Autodesk Fusion 360 part; units mm, degrees
sketch "Sketch1" plane through (0, 0, 0) normal (0, 0, 1) x (1, 0, 0)
  circle A0 centre (0, 0) radius 5.45
  line L0 (0, 7.5) -> (0, -6)
  line L1 (-1.5, 5.2395) -> (-1.5, 3.45)
  line L2 (-1.5, 3.45) -> (1.5, 3.45)
  line L3 (1.5, 3.45) -> (1.5, 5.2395)
  circle A1 centre (0, 0) radius 3.2
  line L4 (-2.0805, -2.4314) -> (2.0805, -2.4314)
  point P0 (0, 5.45)
  dimension "d1" = 10.9
  dimension "d2" = 2
  dimension "d3" = 3
  dimension "d4" = 6.4
  dimension "d5" = 4.161
extrude "Extrude1" add sketch "Sketch1" along normal blind 15
extrude "Extrude2" add sketch "Sketch1" against normal blind 12 contours A0 L0 L2 L3 A1 | A0 L0 L2 L3 | A0 L0 L1 L2 A1 | A0 L0 L1 L2 | L0 A1 L4 | L0 A1 L4 picked at (-0.1505, -2.9331) picked at (0.1518, 1.312)
extrude "Extrude3" cut sketch "Sketch1" against normal blind 10 from surface at 15 contours A0 L0 L2 L3 | A0 L0 L1 L2
Geometry check sheet. Reference: the model listing, model coordinates, mm. A direction names the side the tool comes from. Give positions to 0.01 mm unless a question says otherwise; leave off trailing zeros. Order: outer loops, then holes, each group sorted by start corner. A loop starts at its lowest first (then second) coordinate and runs counter-clockwise, first axis right, second up. Notation, with made-up numbers: (-4.5, 75.5) - (6.5, 75.5) arc R15 ccw to (6.5, 79.5) - close; hole circle Ø8 at (2, 65.5). An arc over 180 degrees is marked (long way). Write item = value, one per line. Start each with the question number.
1) Draft check along Y on faces 4 (the cylindrical face through (-2.982, 1.16, -5.916)), 5 (the flat face through (1, 0, -12)), 6 (the flat face through (0, 3.45, 10)), 7 (the flat face through (-1, 0, 0)). Enter one of: released by +Y, released by -Y, zero draft, split by the parting line, or undercut.
2) Scan lines: L1, parallel to X at y = 0, z = -4; L2, parallel to Z at x = 1, y = -2.5; L3, parallel to Y at x = 1.25, z = -7.5. Record each from-to range of solid material in increasing order.
3) Section check A-A (y = 0). Enter the section's corners in (x, z).
4) Section check D-D (x = 3.25). Enter the section's corners in (y, z), then the cut area to 3 significant figures.
5) Gauge pin test, flat ends, axial feed: pin 1 Ø2.5 at (x, z) = (1.5, -5) entering from -Y; pin 2 Ø1.5 at (y, z) = (4, 10.5) entering from -X; pin 3 Ø1.6 at (x, y) = (0.5, 4.5) entering from +Z. Record the tip position at first contact, or that the pin passes through.
6) Access from +Z, -Z, +X, -X, +Y, -Y to the whole of each face (thin tool, end or side, straight path). Record for faces 1 (the cylindrical face through (2.515, -4.835, 1.689)), 2 (the flat face through (0, 0, -6)), 3 (the flat face through (-1.5, 4, 10)).
7) Section check C-C (z = 10.5). Enter the section's corners in (x, y), then the cut area to 3 significant figures.
Geometry check:
q1.face_4 = undercut
q1.face_5 = zero draft
q1.face_6 = released by +Y
q1.face_7 = undercut
q2.L1 = -5.45 to -3.2, 0 to 5.45
q2.L2 = 0 to 15
q2.L3 = -5.3 to -2.95, -2.43 to 5.3
q3.outline = (-5.45, -12) - (-3.2, -12) - (-3.2, 0) - (0, 0) - (0, -12) - (5.45, -12) - (5.45, 15) - (-5.45, 15) - close
q4.outline = (-4.37, -12) - (4.37, -12) - (4.37, 15) - (-4.37, 15) - close
q4.area = 236 mm2
q5.pin_1 = -5.44
q5.pin_2 = -4.37
q5.pin_3 = 5
q6.face_1 = +Z, -Z
q6.face_2 = -Z
q6.face_3 = +Z, +Y
q7.outline = (-1.5, 3.45) - (-1.5, 5.24) arc R5.45 ccw (long way) to (1.5, 5.24) - (1.5, 3.45) - close
q7.area = 87.5 mm2
